from build123d import *

# Parameters (mm, degrees)
BOSS_EXTRUDE1_DEPTH     = 19.05
F_6_CLEARANCE_HOLE1_D   = 3.7973
FILLET1_R               = 3.175
E_0_25_DIAMETER_HOLE1_D = 3.2639
E_0_25_DIAMETER_HOLE2_D = 3.2639


with BuildPart() as part:
    # Sketch1 → Boss-Extrude1 (new body)
    with BuildSketch(Plane.XY):
        with BuildLine():
            Line((-0.10876362, 5.907615883), (6.17773638, 16.796153285))
            Line((6.17773638, 16.796153285), (8.927367037, 15.208653285))
            Line((8.927367037, 15.208653285), (3.739497694, 6.223))
            Line((3.739497694, 6.223), (5.499261314, 3.175))
            ThreePointArc((5.499261314, 3.175), (3.175, -5.499261314), (-5.499261314, -3.175))
            Line((-5.499261314, -3.175), (-7.259024935, -0.127))
            Line((-7.259024935, -0.127), (-17.63476362, -0.127))
            Line((-17.63476362, -0.127), (-17.63476362, 3.048))
            Line((-17.63476362, 3.048), (-5.06176362, 3.048))
            Line((-5.06176362, 3.048), (-0.10876362, 5.907615883))
        make_face()
    extrude(amount=BOSS_EXTRUDE1_DEPTH)

    # #6 Clearance Hole1 (through all)
    with Locations(Plane(origin=(0, 0, 0), x_dir=(-1, 0, 0), z_dir=(0, 0, -1))):
        with Locations((0, 0)):
            Hole(F_6_CLEARANCE_HOLE1_D / 2)

    # Fillet1
    fillet1_edges = [part.edges().sort_by_distance(p)[0] for p in [
        (3.739497694, 6.223, 9.525),
        (-7.259024935, -0.127, 9.525),
    ]]
    fillet(fillet1_edges, radius=FILLET1_R)

    # E (0.25) Diameter Hole1 (through all)
    with Locations(Plane(origin=(0.109985226, -0.0635, 0), x_dir=(0, 0, -1), z_dir=(0.86602540378444, -0.49999999999999784, 0))):
        with Locations((-4.7625, 13.36343783), (-14.2875, 13.36343783)):
            Hole(E_0_25_DIAMETER_HOLE1_D / 2)

    # E (0.25) Diameter Hole2 (through all)
    with Locations(Plane(origin=(-13.36343783, -0.127, 14.2875), x_dir=(-1, 0, 0), z_dir=(0, -1, 0))):
        with Locations((0, 0), (0, 9.525)):
            Hole(E_0_25_DIAMETER_HOLE2_D / 2)


solid = part.part
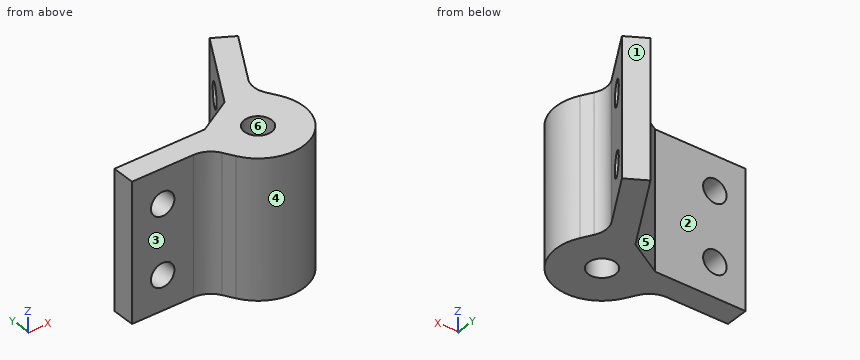
Geometry check sheet. Reference: the model listing, model coordinates, mm. Face numbers are marked on the shaded views. A direction names the side the tool comes from. Round coordinates to 2 decimals unless told otherwise and drop trailing zeros. Write each loop counter-clockwise with the first axis right and the second up, starting at its lowest first coordinate (ties: lowest second). Pieces come first, ordered by that corner, then holes. Notation, with made-up numbers: (-20, 85.25) - (-6, 85.25) arc R14 ccw to (-6, 105.25) - close; hole circle Ø1 at (-36, 87.5). An arc over 180 degrees is marked (long way). One line per item, written item: value.
1. Set-up check for the marked faces 1, 2 and 3: record each of +Z, -Z, +X, -X, +Y, -Y from which the full face is reachable in a straight line by a thin tool's end or side.
The answers:
face 1: +Z, -Z, +X, +Y
face 2: +Z, -Z, -X, +Y
face 3: +Z, -Z, -X, -Y
2. Cross-section at B-B on x = 0.5. Record the boundary of the cut face in (y, z).
The answers:
outline: (-6.33, 0) - (-1.83, 0) - (-1.83, 19.05) - (-6.33, 19.05) - close; (1.83, 0) - (6.96, 0) - (6.96, 19.05) - (1.83, 19.05) - close
3. Depth check by flat-ended pin: pin 1 Ø5 at (x, z) = (-7, 13) entering from -Y; pin 2 Ø5 at (x, z) = (-13.36, 14.29) entering from +Y; pin 3 Ø5 at (x, z) = (-13, 7) entering from -Y. Enter the tip coordinate at first touch or a pass-through.
The answers:
pin 1: stops at y = -4.48
pin 2: stops at y = 3.05
pin 3: stops at y = -0.13
4. Cross-section at D-D on x = -13.5. Record the boundary of the cut face in (y, z), and give its area (3 significant figures).
The answers:
outline: (-0.13, 0) - (3.05, 0) - (3.05, 3.14) - (-0.13, 3.14) - close; (-0.13, 6.39) - (3.05, 6.39) - (3.05, 12.66) - (-0.13, 12.66) - close; (-0.13, 15.91) - (3.05, 15.91) - (3.05, 19.05) - (-0.13, 19.05) - close
area: 39.8 mm^2
5. Scan lines: L1, parallel to X at y = 1.25, z = 6; L2, parallel to Y at x = 0.75, z = 10.25; L3, parallel to Y at x = 6.5, z = 13.75. Record each from-to range of solid material in increasing order.
The answers:
L1: x = -17.63 to -14.43, -12.3 to -1.43, 1.43 to 6.23
L2: y = -6.31 to -1.74, 1.74 to 7.4
L3: y = 13.46 to 16.61
6. Cross-section at A-A on z = 5.5. Give the number of separate pieces and of enclosed holes in the cut face, and give its area (3 significant figures).
The answers:
separate pieces: 3
enclosed holes: 1
area: 167 mm^2
7. Mould release check, pull along X, two halves, no side actions. Record for the marked faces 4, 5 and 6: released by +X, released by -X, zero draft, split by the parting line, or undercut.
The answers:
face 4: split by the parting line
face 5: released by -X
face 6: undercut
